Part print with two shaded views. Sizes in mm from the minimum x, y, z corner. Round coordinates to 2 decimals unless told otherwise and drop trailing zeros. Loops run counter-clockwise (first coordinate to the right, second up) from the corner with the lowest first, then second, coordinate; pieces in that order, holes last. Notation, with made-up numbers: M 21.5,9.25 L 49.5,9.25 A16 cw 49.5,27.25 Z; hole C -2,69.5 d4. An arc over 180 degrees is marked long. Put each result on its own line as item: value. Start each with the question number.
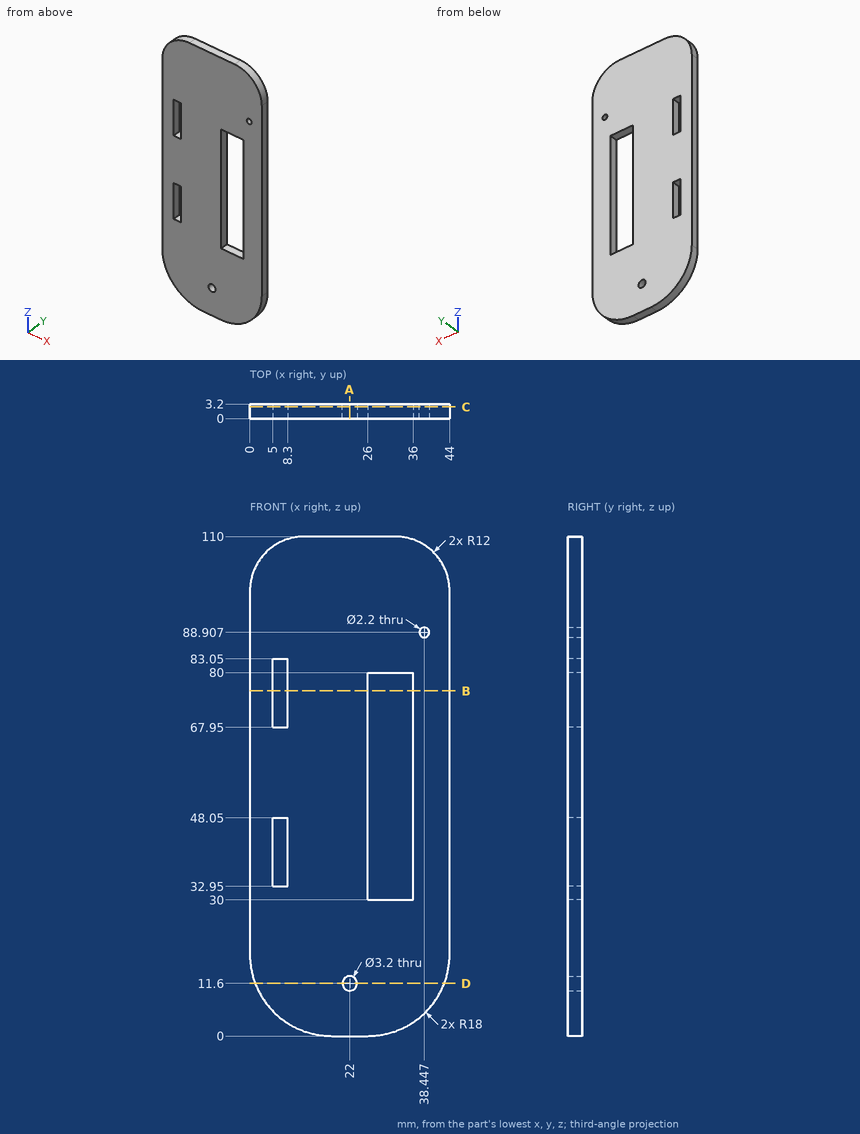
(1) Cut at A-A on x = 22. List the corners of the cut face in (y, z).
(2) Cut at D-D on z = 11.6. List the corners of the cut face in (x, y).
(3) Cut at C-C on y = 2.55. List the corners of the cut face in (x, z).
(4) Flat gauge pins, fed straight in: pin 1 Ø1.6 at (x, y) = (7.5, 2.5) entering from +Z (1 decimal); pin 2 Ø1 at (x, y) = (36, 1.5) entering from +Z; pin 3 Ø4 at (x, z) = (23.5, 23) entering from -Y; pin 4 Ø1 at (x, y) = (7, 2) entering from -Z. Where does each tip first touch, or does it go through?
(5) Drill centre lines: line 1 along Z through (x, y) = (7, 1.1); line 2 along X through (y, z) = (0.75, 75); line 3 along X through (y, z) = (1.2, 32). Where is each one in solid material? Low to high.
(6) Cut at B-B on z = 76. List the corners of the cut face in (x, y).
Taken from the geometry:
1. outline: M 0,0 L 3.2,0 L 3.2,10 L 0,10 Z; M 0,13.2 L 3.2,13.2 L 3.2,110 L 0,110 Z
2. outline: M 1.18,0 L 20.4,0 L 20.4,3.2 L 1.18,3.2 Z; M 23.6,0 L 42.82,0 L 42.82,3.2 L 23.6,3.2 Z
3. outline: M 0,18 A18 ccw 18,0 L 26,0 A18 ccw 44,18 L 44,98 A12 ccw 32,110 L 12,110 A12 ccw 0,98 Z; hole M 5,32.95 L 8.3,32.95 L 8.3,48.05 L 5,48.05 Z; hole M 5,67.95 L 8.3,67.95 L 8.3,83.05 L 5,83.05 Z; hole C 22,11.6 d3.2; hole M 26,30 L 36,30 L 36,80 L 26,80 Z; hole C 38.45,88.91 d2.2
4. pin 1: z = 109.4
4. pin 2: z = 109.48
4. pin 3: y = 0
4. pin 4: z = 3.38
5. line 1: 3.75 to 32.95, 48.05 to 67.95, 83.05 to 108.91
5. line 2: 0 to 5, 8.3 to 26, 36 to 44
5. line 3: 0 to 26, 36 to 44
6. outline: M 0,0 L 5,0 L 5,3.2 L 0,3.2 Z; M 8.3,0 L 26,0 L 26,3.2 L 8.3,3.2 Z; M 36,0 L 44,0 L 44,3.2 L 36,3.2 Z
